from build123d import *

# Parameters (mm, degrees)
F0_R          = 10
F1_DEPTH      = 200
F1_DEPTH_BACK = 200
F2_W          = 16
F2_H          = 16
F3_DEPTH      = 25


with BuildPart() as f1:
    # F0 (on Front) → F1 (new body, two sides)
    with BuildSketch(Plane.XZ) as f1_sk:
        Circle(F0_R)
    extrude(amount=F1_DEPTH)
    extrude(f1_sk.sketch, amount=-F1_DEPTH_BACK)

    # F2 (on Top) → F3 (cut)
    with BuildSketch(Plane.XY):
        Rectangle(F2_W, F2_H)
    extrude(amount=-F3_DEPTH, mode=Mode.SUBTRACT)


solid = f1.part
Work out the finished part from the listing and answer in its coordinate system (mm). A direction names the side the tool comes from. Round coordinates to 2 decimals unless told otherwise and drop trailing zeros. Loops run counter-clockwise (first coordinate to the right, second up) from the corner with the lowest first, then second, coordinate; pieces in that order, holes last. Notation, with made-up numbers: (50, 36.25) - (66, 36.25) arc R33 ccw to (66, 70.25) - close; hole circle Ø10 at (71.5, 67.25). An arc over 180 degrees is marked (long way). One line per item, written item: value.
Q1. Find section C-C on z = 6.5. Give the vertices of the cut face in (x, y).
Check values:
outline: (-7.6, -200) - (7.6, -200) - (7.6, 200) - (-7.6, 200) - close
Q2. For faces 4 (the flat face through (0, 0, 0)), 5 (the cylindrical face through (5.38, -2.8, 8.43)), determine the directions among +Z, -Z, +X, -X, +Y, -Y from which every point of the face is accessible in a straight line to the end or side of a thin tool.
Check values:
face 4: -Z
face 5: +Y, -Y
Q3. Straight lines are drawn through the part: probe 1 along Y at (x, z) = (6, -1); probe 2 along Z at (x, y) = (-0.75, 78); probe 3 along X at (y, z) = (-14, -1). For each, find the intervals that lie inside material, in ascending order.
Check values:
probe 1: -200 to -8, 8 to 200
probe 2: -9.97 to 9.97
probe 3: -9.95 to 9.95
Q4. Each of these flat-tipped pins is pushed along its axis until it touches: pin 1 Ø1 at (y, z) = (21.5, 4) entering from +X; pin 2 Ø5 at (x, y) = (4.5, -20.5) entering from +Z; pin 3 Ø6.5 at (y, z) = (3, -4) entering from +X; pin 4 Ø1 at (x, y) = (-0.5, 158.5) entering from +Z. Where does it stop, or does it pass through?
Check values:
pin 1: x = 9.37
pin 2: z = 9.8
pin 3: x = 9.97
pin 4: z = 10
Q5. Find section A-A on x = 0. Give the vertices of the cut face in (y, z).
Check values:
outline: (-200, -10) - (-8, -10) - (-8, 0) - (8, 0) - (8, -10) - (200, -10) - (200, 10) - (-200, 10) - close
Q6. The mould has two halves that part along Y. Classify faces 1 (the flat face through (0, 200, 0)), 2 (the flat face through (0, -8, -5)), 3 (the flat face through (0, -200, 0)): +Y half, -Y half, draft (parallel to the pull), parting line (faces both ways), or undercut.
Check values:
face 1: +Y half
face 2: undercut
face 3: -Y half
Q7. Find section B-B on y = -81.5. Give the vertices of the cut face in (x, z).
Check values:
outline: circle Ø20 at (0, 0)
